Check sheet for the drawn part. Datum: minimum x, y, z corner. Units: mm. A direction names the side the tool comes from. Give positions to 0.01 mm unless a question says otherwise; leave off trailing zeros. Write each loop counter-clockwise with the first axis right and the second up, starting at its lowest first coordinate (ties: lowest second). Pieces come first, ordered by that corner, then holes. Notation, with made-up numbers: M -1,51.25 L 32,51.25 A18 ccw 32,57.25 Z; hole C -38.75,23 d1. An arc over 180 degrees is marked long. Write item = value, one per line.
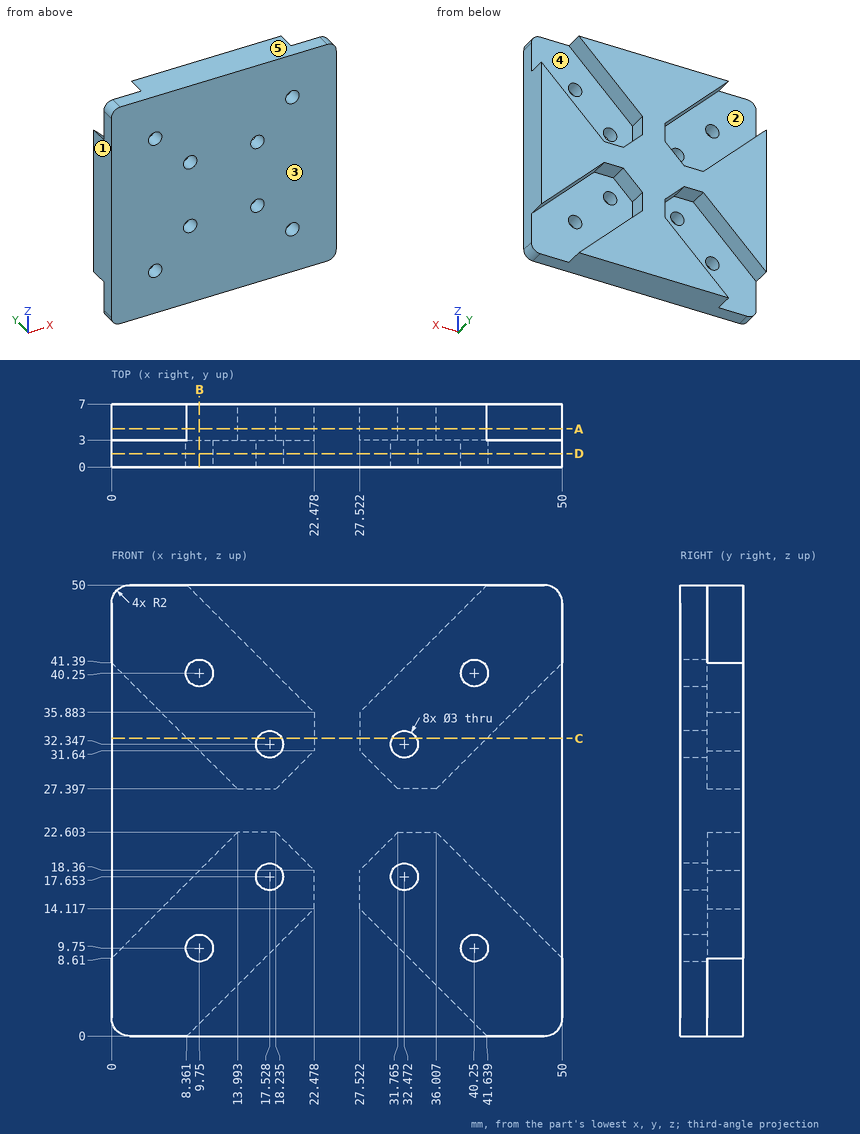
1) Cross-section at B-B on x = 9.75. Record the boundary of the cut face in (y, z), plus the area to 3 significant figures.
From the geometry:
outline = M 0,0 L 7,0 L 7,1.39 L 3,1.39 L 3,8.25 L 0,8.25 Z; M 0,11.25 L 3,11.25 L 3,18.36 L 7,18.36 L 7,31.64 L 3,31.64 L 3,38.75 L 0,38.75 Z; M 0,41.75 L 3,41.75 L 3,48.61 L 7,48.61 L 7,50 L 0,50 Z
area = 196 mm^2
2) Cross-section at A-A on y = 4.25. Record the boundary of the cut face in (x, z) (1 decimal), plus the area to 3 significant figures.
From the geometry:
outline = M 0,8.6 L 14,22.6 L 18.2,22.6 L 22.5,18.4 L 22.5,14.1 L 8.4,0 L 41.6,0 L 27.5,14.1 L 27.5,18.4 L 31.8,22.6 L 36,22.6 L 50,8.6 L 50,41.4 L 36,27.4 L 31.8,27.4 L 27.5,31.6 L 27.5,35.9 L 41.6,50 L 8.4,50 L 22.5,35.9 L 22.5,31.6 L 18.2,27.4 L 14,27.4 L 0,41.4 Z
area = 1,290 mm^2
3) Cross-section at C-C on z = 33. Record the boundary of the cut face in (x, y), plus the area to 3 significant figures.
From the geometry:
outline = M 0,0 L 16.18,0 L 16.18,3 L 8.39,3 L 8.39,7 L 0,7 Z; M 18.88,0 L 31.12,0 L 31.12,3 L 27.52,3 L 27.52,7 L 22.48,7 L 22.48,3 L 18.88,3 Z; M 33.82,0 L 50,0 L 50,7 L 41.61,7 L 41.61,3 L 33.82,3 Z
area = 221 mm^2
4) Tool access check on the marked faces 4 and 5. Record the directions out of +Z, -Z, +X, -X, +Y, -Y that give a thin tool (end or side, any length) a straight path to the whole face; none if there is none.
From the geometry:
face_4 = +Y
face_5 = +Z, +X, -X, +Y, -Y
5) Material ranges on probe 1 along X at (y, z) = (0.75, 32.5); probe 2 along Z at (x, y) = (17.5, 2.25); probe 3 along X at (y, z) = (4, 20.5), recorded low to high. Write a range as from..to.
From the geometry:
probe_1 = 0..16.04, 19.02..30.98, 33.96..50
probe_2 = 0..16.15, 19.15..30.85, 33.85..50
probe_3 = 0..11.89, 20.34..29.66, 38.11..50
6) Cross-section at D-D on y = 1.5. Count the separate pieces of the cut face and the enclosed holes in it, plus the area to 3 significant figures.
From the geometry:
separate_pieces = 1
enclosed_holes = 8
area = 2,440 mm^2
7) Depth check by flat-ended pin: P1, Ø6.5, axis at x = 40.5, z = 41.5, coming from the +Y side. Enter the tip coordinate at first touch or a pass-through.
From the geometry:
P1 = 3
8) Draft check along X on the marked faces 1, 2 and 3. Enter one of: +X half, -X half, draft (parallel to the pull), parting line (faces both ways), or undercut.
From the geometry:
face_1 = -X half
face_2 = undercut
face_3 = draft
